CAD build for the part. Positions are in the model's coordinates, mm. Round coordinates to 2 decimals unless told otherwise and drop trailing zeros. Loops run counter-clockwise (first coordinate to the right, second up) from the corner with the lowest first, then second, coordinate; pieces in that order, holes last.
```python
from build123d import *

# Parameters (mm, degrees)
SKETCH1_R             = 3.379999993
SKETCH1_R_2           = 3.379999996
SKETCH1_R_3           = 3.379999998
SKETCH1_R_4           = 1.13
SKETCH1_R_5           = 3.38
SKETCH1_R_6           = 26.035
SKETCH1_R_7           = 1.663100761
BOSS_EXTRUDE1_DEPTH   = 2.54
F_4_40_TAPPED_HOLE1_D = 2.2606
FILLET1_R             = 1


with BuildPart() as part:
    # Sketch1 → Boss-Extrude1 (new body)
    with BuildSketch(Plane.XY):
        Polygon((93.726, 0), (16.997849999, 0), (0, -16.997849999), (0, -93.726000007), (11, -93.726000007), (11, -119.126000007), (0, -119.126000007), (0, -195.854150007), (16.997849999, -212.852000007), (93.726000007, -212.852000007), (93.726000007, -201.852000007), (119.126000007, -201.852000007), (119.126000007, -212.852000007), (195.854150007, -212.852000007), (212.852000007, -195.854150007), (212.852000007, -119.126), (201.852000007, -119.126), (201.852000007, -93.726), (212.852000007, -93.726), (212.852000007, -16.997849999), (195.854150007, 0), (119.126, 0), (119.126, -11), (93.726, -11), align=None)
        with Locations((30.226, -208.026000005)):
            Circle(SKETCH1_R, mode=Mode.SUBTRACT)
        with Locations((4.825999998, -182.626000003)):
            Circle(SKETCH1_R_2, mode=Mode.SUBTRACT)
        with Locations((55.626, -208.026000005)):
            Circle(SKETCH1_R, mode=Mode.SUBTRACT)
        with Locations((81.026, -208.026000005)):
            Circle(SKETCH1_R, mode=Mode.SUBTRACT)
        with Locations((4.825999998, -157.226000003)):
            Circle(SKETCH1_R_2, mode=Mode.SUBTRACT)
        with Locations((4.825999998, -131.826000003)):
            Circle(SKETCH1_R_2, mode=Mode.SUBTRACT)
        with Locations((131.826, -208.026000005)):
            Circle(SKETCH1_R, mode=Mode.SUBTRACT)
        with Locations((157.226, -208.026000005)):
            Circle(SKETCH1_R, mode=Mode.SUBTRACT)
        with Locations((182.626, -208.026000005)):
            Circle(SKETCH1_R, mode=Mode.SUBTRACT)
        with Locations((208.026000002, -182.626000003)):
            Circle(SKETCH1_R_3, mode=Mode.SUBTRACT)
        with Locations((208.026000002, -157.226000003)):
            Circle(SKETCH1_R_3, mode=Mode.SUBTRACT)
        with Locations((208.026000002, -131.826000003)):
            Circle(SKETCH1_R_3, mode=Mode.SUBTRACT)
        with Locations((4.825999998, -81.026000003)):
            Circle(SKETCH1_R_2, mode=Mode.SUBTRACT)
        with Locations((4.825999998, -55.626000003)):
            Circle(SKETCH1_R_2, mode=Mode.SUBTRACT)
        with Locations((81.026000003, -89.00415)):
            Circle(SKETCH1_R_4, mode=Mode.SUBTRACT)
        with Locations((4.825999998, -30.226000003)):
            Circle(SKETCH1_R_2, mode=Mode.SUBTRACT)
        with Locations((30.226, -4.826000001)):
            Circle(SKETCH1_R_5, mode=Mode.SUBTRACT)
        with Locations((81.026000003, -38.20415)):
            Circle(SKETCH1_R_4, mode=Mode.SUBTRACT)
        with Locations((55.626, -4.826000001)):
            Circle(SKETCH1_R_5, mode=Mode.SUBTRACT)
        with Locations((81.026, -4.826000001)):
            Circle(SKETCH1_R_5, mode=Mode.SUBTRACT)
        with Locations((131.826000003, -89.00415)):
            Circle(SKETCH1_R_4, mode=Mode.SUBTRACT)
        with Locations((106.426000003, -63.60415)):
            Circle(SKETCH1_R_6, mode=Mode.SUBTRACT)
        with Locations((208.026000002, -81.026000003)):
            Circle(SKETCH1_R_3, mode=Mode.SUBTRACT)
        with Locations((208.026000002, -55.626000003)):
            Circle(SKETCH1_R_3, mode=Mode.SUBTRACT)
        with Locations((131.826000003, -38.20415)):
            Circle(SKETCH1_R_4, mode=Mode.SUBTRACT)
        with Locations((131.826, -4.826000001)):
            Circle(SKETCH1_R_5, mode=Mode.SUBTRACT)
        with Locations((157.226, -4.826000001)):
            Circle(SKETCH1_R_5, mode=Mode.SUBTRACT)
        with Locations((171.093920154, -28.877267348)):
            Circle(SKETCH1_R_7, mode=Mode.SUBTRACT)
        with Locations((208.026000002, -30.226000003)):
            Circle(SKETCH1_R_3, mode=Mode.SUBTRACT)
        with Locations((182.626, -4.826000001)):
            Circle(SKETCH1_R_5, mode=Mode.SUBTRACT)
    extrude(amount=BOSS_EXTRUDE1_DEPTH)

    # #4-40 Tapped Hole1 (through all)
    with Locations(Plane(origin=(81.026000003, -38.20415, 2.54), x_dir=(1, 0, 0), z_dir=(0, 0, 1))):
        with Locations((0, 0), (50.8, 0), (50.8, -50.8), (0, -50.8)):
            Hole(F_4_40_TAPPED_HOLE1_D / 2)

    # Fillet1
    fillet1_edges = [part.edges().sort_by_distance(p)[0] for p in [
        (0, -119.126000007, 1.27),
        (11, -119.126000007, 1.27),
        (11, -93.726000007, 1.27),
        (0, -93.726000007, 1.27),
        (93.726, 0, 1.27),
        (93.726, -11, 1.27),
        (119.126, -11, 1.27),
        (119.126, 0, 1.27),
        (212.852000007, -93.726, 1.27),
        (201.852000007, -93.726, 1.27),
        (201.852000007, -119.126, 1.27),
        (212.852000007, -119.126, 1.27),
        (119.126000007, -212.852000007, 1.27),
        (119.126000007, -201.852000007, 1.27),
        (93.726000007, -201.852000007, 1.27),
        (93.726000007, -212.852000007, 1.27),
    ]]
    fillet(fillet1_edges, radius=FILLET1_R)


solid = part.part
```
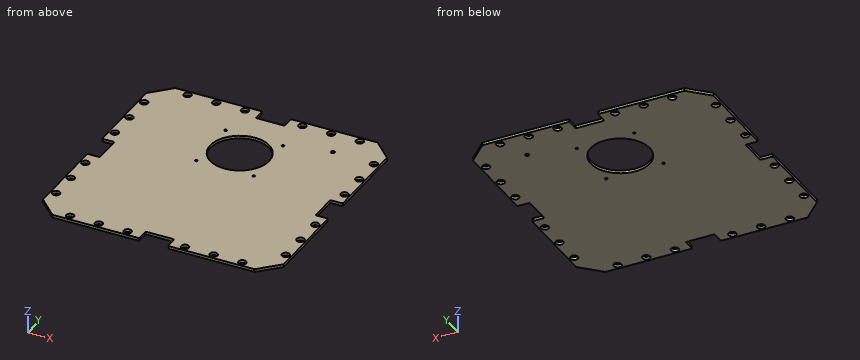
Item 1: Cut at A-A, the plane y = -42.5. Give the cut face in (x, z).
Answers follow:
outline: (0, 0) - (91.18, 0) - (91.18, 2.54) - (0, 2.54) - close; (121.67, 0) - (212.85, 0) - (212.85, 2.54) - (121.67, 2.54) - close
Item 2: Cut at D-D, the plane z = 1.35. State how many separate pieces and enclosed holes the cut face has, plus the area to 3 significant figures.
Answers follow:
separate pieces: 1
enclosed holes: 30
area: 40,600 mm2
Item 3: Cut at B-B, the plane x = 106. Give the cut face in (y, z).
Answers follow:
outline: (-201.85, 0) - (-89.64, 0) - (-89.64, 2.54) - (-201.85, 2.54) - close; (-37.57, 0) - (-11, 0) - (-11, 2.54) - (-37.57, 2.54) - close
Item 4: Probe line 1 (Y direction, x = 183, z = 2); line 2 (Y direction, x = 107, z = 0.6); line 3 (Y direction, x = 79.5, z = 0.45). List the from-to ranges inside material, lowest first.
Answers follow:
line 1: y = -212.85 to -211.39, -204.67 to -8.19, -1.47 to 0
line 2: y = -201.85 to -89.63, -37.58 to -11
line 3: y = -212.85 to -211.04, -205.01 to -7.84, -1.81 to 0
Item 5: Cut at C-C, the plane x = 55.5. Give the cut face in (y, z), plus the area to 3 significant figures.
Answers follow:
outline: (-212.85, 0) - (-211.4, 0) - (-211.4, 2.54) - (-212.85, 2.54) - close; (-204.65, 0) - (-8.2, 0) - (-8.2, 2.54) - (-204.65, 2.54) - close; (-1.45, 0) - (0, 0) - (0, 2.54) - (-1.45, 2.54) - close
area: 506 mm2
Item 6: Flat gauge pins, fed straight in: P1, Ø4, axis at x = 4.826, y = -55.626, coming from the +Z side; P2, Ø0.8, axis at x = 104.5, z = 1, coming from the -Y side; P3, Ø0.8, axis at x = 102, z = 0.5, coming from the +Y side; P4, Ø1.3, axis at y = -7.5, z = 1.5, coming from the -X side. Where does each tip first touch, or does it go through?
Answers follow:
P1: passes through
P2: stops at y = -201.85
P3: stops at y = -11
P4: stops at x = 8.85
